```python
from build123d import *

# Parameters (mm, degrees)
F0_R          = 19.8744550468
F1_DEPTH      = 37.0859950781
F1_DEPTH_BACK = 38.5084822774
F3_D          = 15
F6_DEPTH      = 19.8722034693
F7_DEPTH      = 16.9176664203
F9_DEPTH      = 25
F11_DEPTH     = 25
F13_D         = 15


with BuildPart() as f1:
    # F0 (on Right) → F1 (new body, two sides)
    with BuildSketch(Plane.YZ) as f1_sk:
        with Locations((-43.2518944144, 28.8682542741)):
            Circle(F0_R)
    extrude(amount=F1_DEPTH)
    extrude(f1_sk.sketch, amount=-F1_DEPTH_BACK)

    # F3 (through all)
    with Locations(Plane(origin=(-38.5084822774, 0, 0), x_dir=(0, -1, 0), z_dir=(-1, 0, 0))):
        with Locations((43.2518944144, 28.8682542741)):
            Hole(F3_D / 2)

    # F4 (on face) → F6 (join)
    with BuildSketch(Plane(origin=(-38.5084822774, 0, 0), x_dir=(0, -1, 0), z_dir=(-1, 0, 0))):
        with BuildLine():
            Line((25.5346700703, 92.9932743311), (25.5346700703, 37.8734708149))
            ThreePointArc((25.5346700703, 37.8734708149), (42.4117718159, 48.7249447694), (60.1451545954, 39.3378160541))
            Line((60.1451545954, 39.3378160541), (60.1451545954, 92.9932743311))
            Line((60.1451545954, 92.9932743311), (25.5346700703, 92.9932743311))
        make_face()
    extrude(amount=-F6_DEPTH)

    # F5 (on face) → F7 (join)
    with BuildSketch(Plane.YZ.offset(37.0859950781)):
        with BuildLine():
            ThreePointArc((-60.0371137261, 39.51017027), (-42.1917249238, 48.7144126948), (-25.4284662629, 37.6613977583))
            Line((-25.4284662629, 37.6613977583), (-25.4284662629, 92.7953794599))
            Line((-25.4284662629, 92.7953794599), (-60.0371137261, 92.7953794599))
            Line((-60.0371137261, 92.7953794599), (-60.0371137261, 39.51017027))
        make_face()
    extrude(amount=-F7_DEPTH)

    # F8 (on face) → F9 (cut)
    with BuildSketch(Plane(origin=(-38.5084822774, 0, 0), x_dir=(0, -1, 0), z_dir=(-1, 0, 0))):
        with BuildLine():
            ThreePointArc((25.5346700703, 75.9382109612), (43.0672230686, 91.7866784097), (60.1451545954, 75.4493411154))
            Line((60.1451545954, 75.4493411154), (60.1451545954, 92.9932743311))
            Line((60.1451545954, 92.9932743311), (25.5346700703, 92.9932743311))
            Line((25.5346700703, 92.9932743311), (25.5346700703, 75.9382109612))
        make_face()
    extrude(amount=-F9_DEPTH, mode=Mode.SUBTRACT)

    # F10 (on face) → F11 (cut)
    with BuildSketch(Plane(origin=(20.1683286577, 0, 0), x_dir=(0, -1, 0), z_dir=(-1, 0, 0))):
        with BuildLine():
            ThreePointArc((25.4284662629, 75.7083371282), (42.6920558049, 91.7887475509), (60.0371137261, 75.7962465286))
            Line((60.0371137261, 75.7962465286), (60.0371137261, 92.7953794599))
            Line((60.0371137261, 92.7953794599), (25.4284662629, 92.7953794599))
            Line((25.4284662629, 92.7953794599), (25.4284662629, 75.7083371282))
        make_face()
    extrude(amount=-F11_DEPTH, mode=Mode.SUBTRACT)

    # F13 (through all)
    with Locations(Plane.YZ.offset(37.0859950781)):
        with Locations((-42.7361378145, 74.4343039762)):
            Hole(F13_D / 2)


solid = f1.part
```
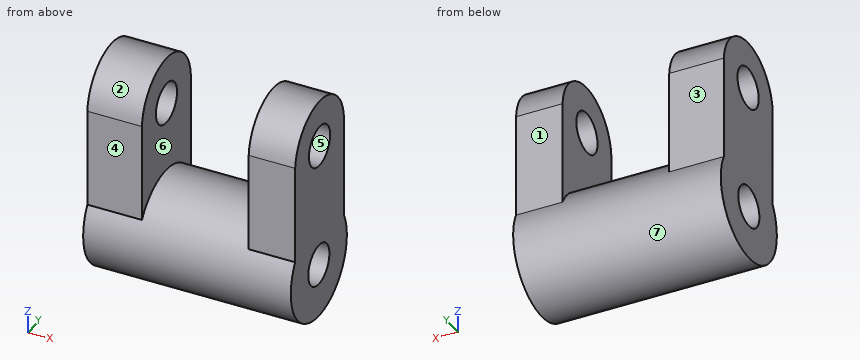
Source: CAD feature listing. Evaluate the final solid. Frame: model axes, mm. Face numbers are marked on the shaded views. A direction names the side the tool comes from. Give positions to 0.01 mm unless a question says otherwise; leave off trailing zeros. Loops run counter-clockwise (first coordinate to the right, second up) from the corner with the lowest first, then second, coordinate; pieces in that order, holes last. Notation, with made-up numbers: (-13, 33) -> (25, 33) arc R22 cw to (25, 65) -> close; hole circle Ø7 at (34.25, 45). An arc over 180 degrees is marked (long way). Use a Markdown table: item, result. Add a question column.
(1) Pull-direction query (Z, two-part tool) for the marked faces 5, 6 and 7; classes: +Z half, -Z half, draft (parallel to the pull), parting line (faces both ways), or undercut.
(2) Section query B-B (z = 72.5). Output: boundary loops of the cut face in (x, y), then the cut area to 3 significant figures.
(3) Section query A-A (y = -44.5). Output: boundary loops of the cut face in (x, z), then the cut area to 3 significant figures.
(4) Section query C-C (x = -30). Output: boundary loops of the cut face in (y, z).
(5) Section query D-D (z = 35). Output: boundary loops of the cut face in (x, y), then the cut area to 3 significant figures.
(6) Ray query, line 1 (X direction, y = -50.5, z = 66); line 2 (Z direction, x = 23, y = -44.5); line 3 (Z direction, x = -30.5, y = -39). Return the intervals inside material, ascending.
(7) First-contact query: pin 1 Ø3 at (x, z) = (-2, 27) entering from -Y; pin 2 Ø18.5 at (x, z) = (30.5, 55.5) entering from +Y; pin 3 Ø1.5 at (x, y) = (4, -48.5) entering from -Z. Flat tips, straight axial feed; report the tip coordinate or a pass-through.
(8) Access query for the marked faces 1, 2, 3 and 4. Directions: +Z, -Z, +X, -X, +Y, -Y. A direction counts if a zero-diameter tool reaches every point of the face in a straight line with its end or side. Return the directions, or none.
Checked values:
| question | item | result |
|---|---|---|
| 1 | face 5 | undercut |
| 1 | face 6 | draft |
| 1 | face 7 | parting line |
| 2 | outline | (-38.51, -60.15) -> (-18.64, -60.15) -> (-18.64, -49.98) -> (-38.51, -49.98) -> close; (-38.51, -35.49) -> (-18.64, -35.49) -> (-18.64, -25.53) -> (-38.51, -25.53) -> close; (20.17, -60.04) -> (37.09, -60.04) -> (37.09, -49.98) -> (20.17, -49.98) -> close; (20.17, -35.49) -> (37.09, -35.49) -> (37.09, -25.43) -> (20.17, -25.43) -> close |
| 2 | area | 740 mm^2 |
| 3 | outline | (-38.51, 9.03) -> (37.09, 9.03) -> (37.09, 21.47) -> (-38.51, 21.47) -> close; (-38.51, 36.26) -> (37.09, 36.26) -> (37.09, 67.14) -> (20.17, 67.14) -> (20.17, 48.7) -> (-18.64, 48.7) -> (-18.64, 67.14) -> (-38.51, 67.14) -> close; (-38.51, 81.72) -> (-18.64, 81.72) -> (-18.64, 91.71) -> (-38.51, 91.71) -> close; (20.17, 81.72) -> (37.09, 81.72) -> (37.09, 91.7) -> (20.17, 91.7) -> close |
| 3 | area | 2,930 mm^2 |
| 4 | outline | (-60.15, 39.34) arc R19.87 ccw (long way) to (-25.53, 37.87) -> (-25.53, 75.94) arc R17.35 ccw to (-60.15, 75.45) -> close; hole circle Ø15 at (-43.25, 28.87); hole circle Ø15 at (-42.74, 74.43) |
| 5 | outline | (-38.51, -62.16) -> (37.09, -62.16) -> (37.09, -47.57) -> (-38.51, -47.57) -> close; (-38.51, -38.93) -> (37.09, -38.93) -> (37.09, -24.35) -> (-38.51, -24.35) -> close |
| 5 | area | 2,210 mm^2 |
| 6 | line 1 | -38.51 to -18.64, 20.17 to 37.09 |
| 6 | line 2 | 9.03 to 21.47, 36.26 to 67.14, 81.72 to 91.7 |
| 6 | line 3 | 9.45 to 22.69, 35.05 to 67.93, 80.94 to 91.36 |
| 7 | pin 1 | y = -63.12 |
| 7 | pin 2 | y = -25.43 |
| 7 | pin 3 | z = 9.51 |
| 8 | face 1 | +Z, +X, -X, +Y |
| 8 | face 2 | +Z, -X |
| 8 | face 3 | +Z, -X, +Y |
| 8 | face 4 | +Z, +X, -X, -Y |
